The listing builds one solid part. Answer for the finished solid, in the listing's coordinates (mm). A direction names the side the tool comes from. Coordinates: 2 decimals unless noted, no trailing zeros. Order: outer loops, then holes, each group sorted by start corner. A loop starts at its lowest first (then second) coordinate and runs counter-clockwise, first axis right, second up. Notation, with made-up numbers: M 43,-28.5 L 56,-28.5 A24 cw 56,-2.5 Z; hole C 76,15 d9. An arc over 180 degrees is marked long. One line per item, written item: value. Start each with the question number.
Q1. For faces 4 (the flat face through (3, 7, 15)), 5 (the flat face through (1, 8.9, 21)), 6 (the flat face through (11, 8.9, 1)), determine the directions among +Z, -Z, +X, -X, +Y, -Y from which every point of the face is accessible in a straight line to the end or side of a thin tool.
Q2. The part is cut by section C-C on z = 6. Give the vertices of the cut face in (x, y).
Q3. The part is cut by section A-A on y = 7. Give the vertices of the cut face in (x, z), then the cut area to 3 significant figures.
Q4. Each of these flat-tipped pins is pushed along its axis until it touches: pin 1 Ø2 at (y, z) = (7, 8.5) entering from +X; pin 2 Ø5 at (x, z) = (10.5, 8) entering from -Y; pin 3 Ø2 at (x, y) = (14, 9) entering from +Z. Where does it stop, or does it pass through?
Q5. The part is cut by section D-D on x = 14.5. Give the vertices of the cut face in (y, z).
Q6. Straight lines are drawn through the part: line 1 along Y through (x, z) = (10, 2.5); line 2 along Y through (x, z) = (7, 4); line 3 along Z through (x, y) = (6.25, 3.5). For each, find the intervals that lie inside material, in ascending order. Write a range as [from, to].
Q7. The part is cut by section B-B on x = 6.5. Give the vertices of the cut face in (y, z).
Q8. Determine the mould class of faces 1 (the cylindrical face through (1.521, 1.141, 26.797)), 2 (the cylindrical face through (15, 7, 1)), 3 (the flat face through (1, 5.1, 21)) for opening direction Z: pulls with the +Z half, pulls with the -Z half, needs draft (parallel to the pull), parting line crosses it, or undercut.
```python
from build123d import *

# Parameters (mm, degrees)
BOX002_W                = 5
BOX002_H                = 3.8
BOX002_DEPTH            = 10
CYLINDER_R              = 1.9
CYLINDER_DEPTH          = 10
ARRAY_X_COUNT           = 2
ARRAY_X_PITCH           = 5
BODY002_PLACEMENT_ANGLE = 90
BOX001_W                = 3
BOX001_H                = 14
BOX001_DEPTH            = 28
FILLET001_R             = 4
PAD_DEPTH               = 2
BOX_W                   = 18
BOX_H                   = 14
BOX_DEPTH               = 3
FILLET_R                = 3


with BuildPart() as between_hole_cube:
    # Box002 → Box002 (new body)
    with BuildSketch(Plane(origin=(0, -1.9, 0), x_dir=(1, 0, 0), z_dir=(0, 0, 1))):
        with Locations((2.5, 1.9)):
            Rectangle(BOX002_W, BOX002_H)
    extrude(amount=BOX002_DEPTH)


with BuildPart() as screw_hole_fusion:
    # Cylinder → Cylinder (new body)
    with BuildSketch(Plane.XY):
        Circle(CYLINDER_R)
    extrude(amount=CYLINDER_DEPTH)

    # Array X: screw hole fusion ×2


with BuildPart() as screw_hole_fusion_1:
    add(screw_hole_fusion.part)
    with Locations(*[(i * ARRAY_X_PITCH, 0, 0) for i in range(1, ARRAY_X_COUNT)]):
        add(screw_hole_fusion.part)

    # Fusion002: union between hole cube
    add(between_hole_cube.part)


with BuildPart() as h_screw_hole_fusion_clone:
    # Body002 base: copy of screw hole fusion
    add(screw_hole_fusion_1.part)


with BuildPart() as h_screw_hole_fusion_clone_1:
    # Body002 placement: moved
    add(h_screw_hole_fusion_clone.part.moved(Location((0, 7, 23.1))).rotate(Axis((0, 7, 23.1), (0, 1, 0)), BODY002_PLACEMENT_ANGLE))


with BuildPart() as hole_fusion:
    # Body001 base: copy of screw hole fusion
    add(screw_hole_fusion_1.part)


with BuildPart() as hole_fusion_1:
    # Body001 placement: moved
    add(hole_fusion.part.moved(Location((8.1, 7, 0))))

    # Fusion001: union h screw hole fusion clone
    add(h_screw_hole_fusion_clone_1.part)


with BuildPart() as bottom_cube_fillet:
    # Box001 → Box001 (new body)
    with BuildSketch(Plane.XY):
        with Locations((1.5, 7)):
            Rectangle(BOX001_W, BOX001_H)
    extrude(amount=BOX001_DEPTH)

    # Fillet001
    fillet001_edges = [bottom_cube_fillet.edges().sort_by_distance(p)[0] for p in [
        (1.5, 0, 28),
        (1.5, 14, 28),
    ]]
    fillet(fillet001_edges, radius=FILLET001_R)


with BuildPart() as triangle_body:
    # Sketch → Pad (new body)
    with BuildSketch(Plane.XZ):
        Polygon((0, 0), (0, 24.03203), (14.854653, 0), align=None)
    extrude(amount=-PAD_DEPTH)


with BuildPart() as part_mirroring:
    # Part__Mirroring: instance of triangle body
    add(triangle_body.part.mirror(Plane(origin=(0, 7, 0), x_dir=(1, 0, 0), z_dir=(0, 1, 0))))


with BuildPart() as bracket_cut:
    # Box → Box (new body)
    with BuildSketch(Plane.XY):
        with Locations((9, 7)):
            Rectangle(BOX_W, BOX_H)
    extrude(amount=BOX_DEPTH)

    # Fillet
    fillet_edges = [bracket_cut.edges().sort_by_distance(p)[0] for p in [
        (18, 0, 1.5),
        (18, 14, 1.5),
    ]]
    fillet(fillet_edges, radius=FILLET_R)

    # Fusion: union bottom cube fillet, Part__Mirroring, triangle body
    add(bottom_cube_fillet.part)
    add(part_mirroring.part)
    add(triangle_body.part)

    # Cut: cut hole fusion
    add(hole_fusion_1.part, mode=Mode.SUBTRACT)


solid = bracket_cut.part
```
Output:
1. face 4: +Z, +X
1. face 5: +X, -X
1. face 6: +Z, -Z
2. outline: M 0,0 L 11.15,0 L 11.15,2 L 3,2 L 3,12 L 11.15,12 L 11.15,14 L 0,14 Z
3. outline: M 0,0 L 6.2,0 L 6.2,3 L 3,3 L 3,16.2 L 0,16.2 Z; M 0,25 L 3,25 L 3,28 L 0,28 Z; M 15,0 L 18,0 L 18,3 L 15,3 Z
3. area: 76.2 mm^2
4. pin 1: stops at x = 3
4. pin 2: stops at y = 0
4. pin 3: stops at z = 3
5. outline: M 0,0 L 5.72,0 L 5.72,3 L 0,3 Z; M 8.28,0 L 14,0 L 14,3 L 8.28,3 Z
6. line 1: y = [0, 5.1], [8.9, 14]
6. line 2: y = [0, 2], [12, 14]
6. line 3: z = [0, 3]
7. outline: M 0,0 L 5.98,0 L 5.98,3 L 2,3 L 2,13.52 L 0,13.52 Z; M 8.02,0 L 14,0 L 14,13.52 L 12,13.52 L 12,3 L 8.02,3 Z
8. face 1: pulls with the +Z half
8. face 2: needs draft
8. face 3: undercut
